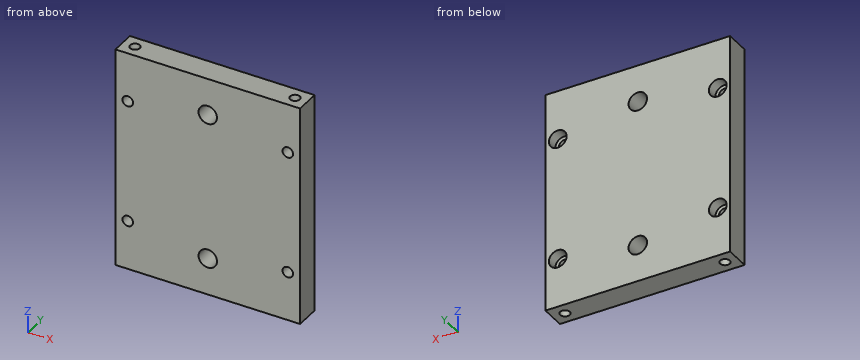
Autodesk Inventor part; units mm, degrees
ref_plane "YZ Plane" through (0, 0, 0) normal (1, 0, 0) x (0, 1, 0)
ref_plane "XZ Plane" through (0, 0, 0) normal (0, 1, 0) x (-1, 0, 0)
ref_plane "XY Plane" through (0, 0, 0) normal (0, 0, 1) x (1, 0, 0)
sketch "Sketch1" plane through (0, 0, 0) normal (0, 1, 0) x (-1, 0, 0)
  line L0 (-37.5, 45) -> (37.5, 45)
  line L1 (37.5, 45) -> (37.5, -45)
  line L2 (37.5, -45) -> (-37.5, -45)
  line L3 (-37.5, -45) -> (-37.5, 45)
  line L4 (-37.5, 45) -> (37.5, -45) construction
  line L5 (37.5, 45) -> (-37.5, -45) construction
  point P0 (0, 0)
  dimension "d0" = 75
  dimension "d1" = 90
extrude "Extrusion1" add sketch "Sketch1" along normal blind 10
sketch "Sketch2" plane through (0, 10, 0) normal (0, 1, 0) x (1, 0, 0)
  line L0 (-37.5, -45) -> (37.5, -45)
  line L1 (37.5, -45) -> (37.5, -25)
  line L2 (37.5, -45) -> (37.5, 45)
  line L3 (37.5, -25) -> (32.5, -25)
  circle A0 centre (32.5, -25) radius 2.15
  line L4 (0, 0) -> (37.5, 0)
  line L5 (-37.5, 45) -> (37.5, 45)
  line L6 (37.5, 45) -> (37.5, 25)
  line L7 (37.5, 45) -> (37.5, -45)
  line L8 (37.5, 25) -> (32.5, 25)
  circle A1 centre (32.5, 25) radius 2.15
  line L9 (0, -45) -> (0, 45)
  line L10 (-37.5, -45) -> (-37.5, -25)
  line L11 (-37.5, -45) -> (-37.5, 45)
  line L12 (-37.5, -25) -> (-32.5, -25)
  circle A2 centre (-32.5, -25) radius 2.15
  line L13 (-37.5, 45) -> (-37.5, 25)
  line L14 (-37.5, 45) -> (-37.5, -45)
  line L15 (-37.5, 25) -> (-32.5, 25)
  circle A3 centre (-32.5, 25) radius 2.15
  point P0 (-37.5, 0)
  dimension "d4" = 20
  dimension "d5" = 5
  dimension "d6" = 4.3
extrude "Extrusion2" cut sketch "Sketch2" against normal blind 10 contours A3 | A2 | A0 | A1
sketch "Sketch3" plane through (0, 10, 0) normal (0, 1, 0) x (1, 0, 0)
  circle A0 centre (32.5, -25) radius 3.61
  circle A1 centre (32.5, -25) radius 2.15
  line L0 (0, 0) -> (29.9913, 0)
  line L1 (-37.5, -45) -> (37.5, -45)
  line L2 (0, -45) -> (0, 45)
  circle A2 centre (32.5, -25) radius 2
  circle A3 centre (32.5, 25) radius 3.61
  circle A4 centre (32.5, 25) radius 2.15
  circle A5 centre (32.5, 25) radius 2
  circle A6 centre (-32.5, -25) radius 3.61
  circle A7 centre (-32.5, -25) radius 2.15
  circle A8 centre (-32.5, -25) radius 2
  circle A9 centre (-32.5, 25) radius 3.61
  circle A10 centre (-32.5, 25) radius 2.15
  circle A11 centre (-32.5, 25) radius 2
  point P0 (-29.9913, 0)
  dimension "d11" = 7.22
  dimension "d14" = 4
extrude "Extrusion3" cut sketch "Sketch3" against normal blind 4.5 contours A0 | A3 | A6 | A9
sketch "Sketch4" plane through (0, 10, 0) normal (0, 1, 0) x (1, 0, 0)
  line L0 (-37.5, -45) -> (37.5, -45)
  line L1 (37.5, -45) -> (0, -45)
  line L2 (0, -45) -> (0, -30)
  circle A0 centre (0, -30) radius 3.75
  line L3 (37.5, 45) -> (-37.5, 45)
  line L4 (-37.5, 45) -> (0, 45)
  line L5 (0, 45) -> (0, 30)
  circle A1 centre (0, 30) radius 3.75
  point P0 (0, 0)
  dimension "d17" = 37.5
  dimension "d18" = 15
  dimension "d19" = 7.5
  dimension "d22" = 37.5
  dimension "d23" = 15
  dimension "d24" = 7.5
extrude "Extrusion5" cut sketch "Sketch4" against normal blind 10
sketch "Sketch7" plane through (0, 10, 0) normal (0, 1, 0) x (1, 0, 0)
  circle A0 centre (0, 30) radius 3.75
sketch "Sketch8" plane through (0, 10, 0) normal (0, 1, 0) x (1, 0, 0)
  circle A0 centre (0, -30) radius 3.75
sketch "Sketch9" plane through (-37.5, 0, 45) normal (0, 0, 1) x (1, 0, 0)
  line L0 (0, 0) -> (0, 10)
  line L1 (0, 5) -> (5, 5)
  circle A0 centre (5, 5) radius 2
  line L2 (75, 0) -> (75, 10)
  line L3 (75, 5) -> (70, 5)
  circle A1 centre (70, 5) radius 2
  point P0 (37.5, 0)
  dimension "d28" = 5
  dimension "d29" = 4
  dimension "d30" = 5
  dimension "d31" = 4
sketch "Sketch10" plane through (37.5, 0, -45) normal (0, 0, -1) x (-1, 0, 0)
  line L0 (0, 0) -> (0, 10)
  line L1 (0, 5) -> (5, 5)
  line L2 (75, 0) -> (75, 10)
  line L3 (75, 5) -> (70, 5)
  circle A0 centre (5, 5) radius 2
  circle A1 centre (70, 5) radius 2
  point P0 (37.5, 0)
  dimension "d32" = 5
  dimension "d33" = 5
  dimension "d34" = 4
  dimension "d35" = 4
extrude "Extrusion6" cut sketch "Sketch10" against normal blind 15
extrude "Extrusion7" cut sketch "Sketch9" against normal blind 15
thread "Thread1"
thread "Thread2"
thread "Thread3"
thread "Thread4"
properties part number "Rb PEEK - Arriba"
The model under review builds one solid part; all positions refer to its coordinate system, in mm. Coordinates: 2 decimals unless noted, no trailing zeros. Loops run counter-clockwise (first coordinate to the right, second up) from the corner with the lowest first, then second, coordinate; pieces in that order, holes last. Notation, with made-up numbers: (66.25, 80.25) -> (84.25, 80.25) arc R26 cw to (84.25, 111.25) -> close; hole circle Ø5 at (-6.75, -40). An arc over 180 degrees is marked (long way). Use a Markdown table: item, result. Add a question column.
1. Clearance check with flat-ended pins moving along their axes: pin 1 Ø3 at (x, y) = (32.5, 5) entering from +Z; pin 2 Ø4.5 at (x, z) = (-32.5, 25) entering from +Y; pin 3 Ø4 at (x, z) = (-32.5, 25) entering from -Y; pin 4 Ø2 at (x, y) = (-32.5, 5.5) entering from -Z. State where each tip first meets the part, or that it passes through.
2. Add section B-B on x = 32.5. Write out the cut boundary in (y, z), plus the area to 3 significant figures.
3. To check wall thickness, follow line 1 (X direction, y = 3, z = -25); line 2 (Z direction, x = 32.5, y = 2.1); line 3 (X direction, y = 8, z = 25). State the ranges of each line that lie inside material, in increasing order.
4. Add section C-C on z = -25. Write out the cut boundary in (x, y), plus the area to 3 significant figures.
5. Add section A-A on y = 1.5. Write out the cut boundary in (x, z), plus the area to 3 significant figures.
6. Add section D-D on y = 8.5. Write out the cut boundary in (x, z).
Returned:
| question | item | result |
|---|---|---|
| 1 | pin 1 | stops at z = 30 |
| 1 | pin 2 | stops at y = 5.5 |
| 1 | pin 3 | passes through |
| 1 | pin 4 | stops at z = -30 |
| 2 | outline | (0, -45) -> (3, -45) -> (3, -30) -> (7, -30) -> (7, -45) -> (10, -45) -> (10, -28.61) -> (5.5, -28.61) -> (5.5, -27.15) -> (0, -27.15) -> close; (0, -22.85) -> (5.5, -22.85) -> (5.5, -21.39) -> (10, -21.39) -> (10, 21.39) -> (5.5, 21.39) -> (5.5, 22.85) -> (0, 22.85) -> close; (0, 27.15) -> (5.5, 27.15) -> (5.5, 28.61) -> (10, 28.61) -> (10, 45) -> (7, 45) -> (7, 30) -> (3, 30) -> (3, 45) -> (0, 45) -> close |
| 2 | area | 668 mm² |
| 3 | line 1 | x = -37.5 to -34.65, -30.35 to 30.35, 34.65 to 37.5 |
| 3 | line 2 | z = -45 to -27.15, -22.85 to 22.85, 27.15 to 45 |
| 3 | line 3 | x = -37.5 to -36.11, -28.89 to 28.89, 36.11 to 37.5 |
| 4 | outline | (-37.5, 0) -> (-34.65, 0) -> (-34.65, 5.5) -> (-36.11, 5.5) -> (-36.11, 10) -> (-37.5, 10) -> close; (-30.35, 0) -> (30.35, 0) -> (30.35, 5.5) -> (28.89, 5.5) -> (28.89, 10) -> (-28.89, 10) -> (-28.89, 5.5) -> (-30.35, 5.5) -> close; (34.65, 0) -> (37.5, 0) -> (37.5, 10) -> (36.11, 10) -> (36.11, 5.5) -> (34.65, 5.5) -> close |
| 4 | area | 638 mm² |
| 5 | outline | (-37.5, -45) -> (37.5, -45) -> (37.5, 45) -> (-37.5, 45) -> close; hole circle Ø4.3 at (-32.5, -25); hole circle Ø4.3 at (-32.5, 25); hole circle Ø7.5 at (0, -30); hole circle Ø7.5 at (0, 30); hole circle Ø4.3 at (32.5, -25); hole circle Ø4.3 at (32.5, 25) |
| 5 | area | 6,600 mm² |
| 6 | outline | (-37.5, -45) -> (37.5, -45) -> (37.5, 45) -> (-37.5, 45) -> close; hole circle Ø7.22 at (-32.5, -25); hole circle Ø7.22 at (-32.5, 25); hole circle Ø7.5 at (0, -30); hole circle Ø7.5 at (0, 30); hole circle Ø7.22 at (32.5, -25); hole circle Ø7.22 at (32.5, 25) |
